```python
from build123d import *

# Parameters (mm, degrees)
SKETCH1_W           = 75
SKETCH1_H           = 10
BOSS_EXTRUDE1_DEPTH = 2.5


with BuildPart() as part:
    # Sketch1 → Boss-Extrude1 (new body)
    with BuildSketch(Plane(origin=(0, 0, 0), x_dir=(0, 0, -1), z_dir=(1, 0, 0))):
        with BuildLine():
            Line((34.2, 5), (37.5, 5))
            Line((37.5, 5), (37.5, 10))
            Line((37.5, 10), (-37.5, 10))
            Line((-37.5, 10), (-37.5, 5))
            Line((-37.5, 5), (-34.2, 5))
            ThreePointArc((-34.2, 5), (-32.5, 6.7), (-30.8, 5))
            Line((-30.8, 5), (30.8, 5))
            ThreePointArc((30.8, 5), (32.5, 6.7), (34.2, 5))
        make_face()
        with BuildLine():
            Line((-37.5, 0), (37.5, 0))
            Line((37.5, 0), (37.5, 5))
            Line((37.5, 5), (34.2, 5))
            ThreePointArc((34.2, 5), (32.5, 3.3), (30.8, 5))
            Line((30.8, 5), (-30.8, 5))
            ThreePointArc((-30.8, 5), (-32.5, 3.3), (-34.2, 5))
            Line((-34.2, 5), (-37.5, 5))
            Line((-37.5, 5), (-37.5, 0))
        make_face()
        with Locations((0, -5)):
            Rectangle(SKETCH1_W, SKETCH1_H)
    extrude(amount=BOSS_EXTRUDE1_DEPTH)


solid = part.part
```
Input: part model. Units: mm. Frame: model coordinates. Coordinates: 2 decimals unless noted, no trailing zeros. Write each loop counter-clockwise with the first axis right and the second up, starting at its lowest first coordinate (ties: lowest second). Pieces come first, ordered by that corner, then holes.
1) Section A-A on z = -32.5. Output: boundary loops of the cut face in (x, y), and give its area (3 significant figures).
2) Section B-B on y = 5. Output: boundary loops of the cut face in (x, z), and give its area (4 significant figures).
3) Material intervals for line 1 along Z through (x, y) = (1.3, 5); line 2 along Y through (x, z) = (0.65, 32.5); line 3 along Z through (x, y) = (1.7, 6), sorted ascending.
4) Mould query, pull axis Y, two halves, no side actions, for faces 1 (the flat face through (2.5, 0, 1)), 2 (the flat face through (1, -10, 1)), 3 (the cylindrical face through (1.23, 4.49, -34.12)), 4 (the cylindrical face through (1.23, 5.65, 30.93)). Classes: pulls with the +Y half, pulls with the -Y half, needs draft (parallel to the pull), parting line crosses it, or undercut.
Check result:
1. outline: (0, -10) - (2.5, -10) - (2.5, 3.3) - (0, 3.3) - close; (0, 6.7) - (2.5, 6.7) - (2.5, 10) - (0, 10) - close
1. area: 41.5 mm2
2. outline: (0, -37.5) - (2.5, -37.5) - (2.5, -34.2) - (0, -34.2) - close; (0, -30.8) - (2.5, -30.8) - (2.5, 30.8) - (0, 30.8) - close; (0, 34.2) - (2.5, 34.2) - (2.5, 37.5) - (0, 37.5) - close
2. area: 170.5 mm2
3. line 1: z = -37.5 to -34.2, -30.8 to 30.8, 34.2 to 37.5
3. line 2: y = -10 to 3.3, 6.7 to 10
3. line 3: z = -37.5 to -33.87, -31.13 to 31.13, 33.87 to 37.5
4. face 1: needs draft
4. face 2: pulls with the -Y half
4. face 3: undercut
4. face 4: undercut
